from build123d import *
from build123d import SkipClean  # not in build123d's __all__

# Parameters (mm, degrees)
F0_W     = 30.5
F0_H     = 44.5
F0_W_2   = 20.5
F0_H_2   = 34.5
F1_DEPTH = 2
F2_DEPTH = 5


with BuildPart() as f1:
    # F0 (on Top) → F1 (new body)
    with BuildSketch(Plane.XY):
        Rectangle(F0_W, F0_H)
        Rectangle(F0_W_2, F0_H_2, mode=Mode.SUBTRACT)
        Rectangle(F0_W_2, F0_H_2)
        with BuildLine():
            ThreePointArc((8.25, 5.6513272777), (9.5524865873, 2.9580398915), (10, 0))
            ThreePointArc((10, 0), (9.5524865873, -2.9580398915), (8.25, -5.6513272777))
            Line((8.25, -5.6513272777), (8.25, -15.25))
            Line((8.25, -15.25), (-8.25, -15.25))
            Line((-8.25, -15.25), (-8.25, -5.6513272777))
            ThreePointArc((-8.25, -5.6513272777), (-10, 0), (-8.25, 5.6513272777))
            Line((-8.25, 5.6513272777), (-8.25, 15.25))
            Line((-8.25, 15.25), (8.25, 15.25))
            Line((8.25, 15.25), (8.25, 5.6513272777))
        make_face(mode=Mode.SUBTRACT)
        with BuildLine():
            ThreePointArc((-8.25, 5.6513272777), (0, 10), (8.25, 5.6513272777))
            Line((8.25, 5.6513272777), (8.25, 15.25))
            Line((8.25, 15.25), (-8.25, 15.25))
            Line((-8.25, 15.25), (-8.25, 5.6513272777))
        make_face()
        with BuildLine():
            Line((8.25, -15.25), (8.25, -5.6513272777))
            ThreePointArc((8.25, -5.6513272777), (0, -10), (-8.25, -5.6513272777))
            Line((-8.25, -5.6513272777), (-8.25, -15.25))
            Line((-8.25, -15.25), (8.25, -15.25))
        make_face()
    extrude(amount=F1_DEPTH)

    # F0 (on Top) → F2 (join)
    with BuildSketch(Plane.XY):
        Rectangle(F0_W_2, F0_H_2)
        with BuildLine():
            ThreePointArc((8.25, 5.6513272777), (9.5524865873, 2.9580398915), (10, 0))
            ThreePointArc((10, 0), (9.5524865873, -2.9580398915), (8.25, -5.6513272777))
            Line((8.25, -5.6513272777), (8.25, -15.25))
            Line((8.25, -15.25), (-8.25, -15.25))
            Line((-8.25, -15.25), (-8.25, -5.6513272777))
            ThreePointArc((-8.25, -5.6513272777), (-10, 0), (-8.25, 5.6513272777))
            Line((-8.25, 5.6513272777), (-8.25, 15.25))
            Line((-8.25, 15.25), (8.25, 15.25))
            Line((8.25, 15.25), (8.25, 5.6513272777))
        make_face(mode=Mode.SUBTRACT)
    with SkipClean():  # cleaning this boolean's faces spoils the solid; the shape is the same uncleaned
        extrude(amount=-F2_DEPTH)


solid = f1.part
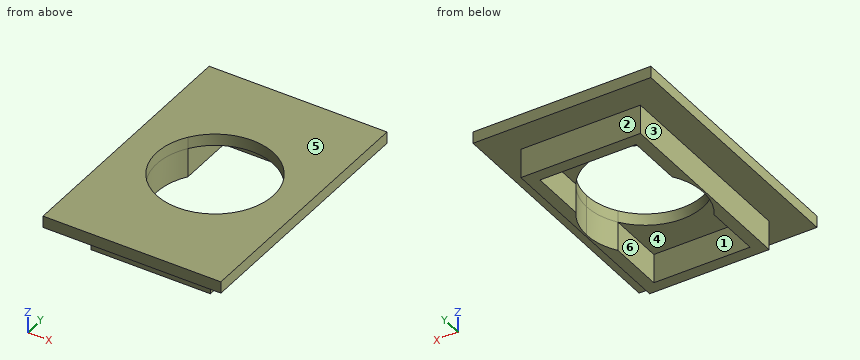
Can you work these out from the model? Positions are in its coordinate system, mm. Face numbers are marked on the shaded views. A direction names the side the tool comes from. Coordinates: 2 decimals unless noted, no trailing zeros. Write each loop counter-clockwise with the first axis right and the second up, starting at its lowest first coordinate (ties: lowest second). Pieces come first, ordered by that corner, then holes. Notation, with made-up numbers: (35.25, 70) - (51.25, 70) arc R17 ccw to (51.25, 94) - close; hole circle Ø9 at (11, 40). An arc over 180 degrees is marked (long way). Return JSON: item names as keys, results as strings. Group by question number.
Item 1: If we section it at D-D (x = -11.5): Write out the boundary of the cut face in (y, z).
Item 2: We'd pull the mould along X, two halves only. Please class the marked faces 1, 2, 3 and 4: pulls with the +X half, pulls with the -X half, needs draft (parallel to the pull), parting line crosses it, or undercut.
Item 3: Please list where these lines run through material, in increasing order: probe 1 along X at (y, z) = (-11.5, -3); probe 2 along Y at (x, z) = (6, -3); probe 3 along X at (y, z) = (0, -0.5).
Item 4: If we section it at C-C (y = -9): Write out the boundary of the cut face in (x, z).
Item 5: Which directions (+Z, -Z, +X, -X, +Y, -Y) give clear straight access to the entire face, cutting with the end or side of a thin tool? Please do the marked faces 5 and 6.
Item 6: If we section it at A-A (x = 6): Write out the boundary of the cut face in (y, z).
Item 7: I'm going to push flat-ended pins straight in: pin 1 Ø1 at (x, z) = (8, -4.5) entering from -Y; pin 2 Ø3 at (x, y) = (-3.5, -10) entering from -Z; pin 3 Ø4 at (y, z) = (-12.5, -3.5) entering from -X. Where does each tip first touch, or does it pass through?
Item 8: If we section it at B-B (z = -4.5): Write out the boundary of the cut face in (x, y).
Return value:
{
 "1": {"outline": "(-22.25, 0) - (22.25, 0) - (22.25, 2) - (-22.25, 2) - close"},
 "2": {"face 1": "undercut", "face 2": "needs draft", "face 3": "pulls with the -X half", "face 4": "undercut"},
 "3": {"probe 1": "x = -10.25 to -8.25, 8.25 to 10.25", "probe 2": "y = -17.25 to -15.25, 15.25 to 17.25", "probe 3": "x = -10.25 to -10, 10 to 10.25"},
 "4": {"outline": "(-15.25, 0) - (-10.25, 0) - (-10.25, -5) - (-8.25, -5) - (-8.25, 0) - (-4.36, 0) - (-4.36, 2) - (-15.25, 2) - close; (4.36, 0) - (8.25, 0) - (8.25, -5) - (10.25, -5) - (10.25, 0) - (15.25, 0) - (15.25, 2) - (4.36, 2) - close"},
 "5": {"face 5": "+Z, +X, -X, +Y, -Y", "face 6": "-Z"},
 "6": {"outline": "(-22.25, 0) - (-17.25, 0) - (-17.25, -5) - (-15.25, -5) - (-15.25, 0) - (-8, 0) - (-8, 2) - (-22.25, 2) - close; (8, 0) - (15.25, 0) - (15.25, -5) - (17.25, -5) - (17.25, 0) - (22.25, 0) - (22.25, 2) - (8, 2) - close"},
 "7": {"pin 1": "stops at y = -17.25", "pin 2": "stops at z = 0", "pin 3": "stops at x = -10.25"},
 "8": {"outline": "(-10.25, -17.25) - (10.25, -17.25) - (10.25, 17.25) - (-10.25, 17.25) - close; hole (-8.25, -15.25) - (8.25, -15.25) - (8.25, -5.65) arc R10 ccw to (8.25, 5.65) - (8.25, 15.25) - (-8.25, 15.25) - (-8.25, 5.65) arc R10 ccw to (-8.25, -5.65) - close"}
}
